The listing builds one solid part. Answer for the finished solid, in the listing's coordinates (mm). A direction names the side the tool comes from. Round coordinates to 2 decimals unless told otherwise and drop trailing zeros. Loops run counter-clockwise (first coordinate to the right, second up) from the corner with the lowest first, then second, coordinate; pieces in that order, holes last. Notation, with made-up numbers: (70.25, -14.75) -> (89.25, -14.75) arc R30 ccw to (89.25, 24.25) -> close; hole circle Ø11 at (80.5, -34). An arc over 180 degrees is marked (long way). Write each question's results on one line, items separated by ' | '. Start each with the question number.
from build123d import *

# Parameters (mm, degrees)
F0_R     = 1
F0_R_2   = 2
F1_DEPTH = 1
F2_R     = 1
F3_DEPTH = 1
F4_SIZE  = 4
F5_SIZE  = 5
F6_R     = 1.5


with BuildPart() as f1:
    # F0 (on Top) → F1 (new body)
    with BuildSketch(Plane.XY):
        with BuildLine():
            Line((-6.25, 2.5), (-6.25, 0))
            ThreePointArc((-6.25, 0), (0, -6.25), (6.25, 0))
            Line((6.25, 0), (6.25, 2.5))
            Line((6.25, 2.5), (-6.25, 2.5))
        make_face()
        with BuildLine():
            ThreePointArc((6.25, 0), (0, -6.25), (-6.25, 0))
            Line((-6.25, 0), (-6.25, 2.5))
            Line((-6.25, 2.5), (-13, 2.5))
            Line((-13, 2.5), (-13, -4.25))
            Line((-13, -4.25), (-10.5, -4.25))
            ThreePointArc((-10.5, -4.25), (-4.25, -10.5), (-10.5, -16.75))
            Line((-10.5, -16.75), (-13, -16.75))
            Line((-13, -16.75), (-13, -32.9777747887))
            Line((-13, -32.9777747887), (13.7, -32.9777747887))
            Line((13.7, -32.9777747887), (13.7, 2.5))
            Line((13.7, 2.5), (6.25, 2.5))
            Line((6.25, 2.5), (6.25, 0))
        make_face()
        with Locations((-10.5, -21)):
            Circle(F0_R, mode=Mode.SUBTRACT)
        with Locations((7.7645713531, -28.9777747887)):
            Circle(F0_R_2, mode=Mode.SUBTRACT)
        with Locations((10.5, -21)):
            Circle(F0_R, mode=Mode.SUBTRACT)
        with Locations((-10.5, 0)):
            Circle(F0_R, mode=Mode.SUBTRACT)
        with Locations((10.5, 0)):
            Circle(F0_R, mode=Mode.SUBTRACT)
    extrude(amount=F1_DEPTH)

    # F2 (on face) → F3 (cut, through all)
    with BuildSketch(Plane.XY.offset(1)):
        Polygon((5.2645713531, -32.9777747887), (-13, -23.5), (-13, -32.9777747887), align=None)
        with BuildLine():
            Line((-13, -16.75), (-13, -18.5))
            Line((-13, -18.5), (8.2, -18.5))
            Line((8.2, -18.5), (8.2, 2.5))
            Line((8.2, 2.5), (-13, 2.5))
            Line((-13, 2.5), (-13, -4.25))
            Line((-13, -4.25), (-10.5, -4.25))
            ThreePointArc((-10.5, -4.25), (-4.25, -10.5), (-10.5, -16.75))
            Line((-10.5, -16.75), (-13, -16.75))
        make_face()
        with Locations((-10.5, 0)):
            Circle(F2_R, mode=Mode.SUBTRACT)
    extrude(amount=-F3_DEPTH, mode=Mode.SUBTRACT)

    # F4
    f4_edges = [f1.edges().sort_by_distance(p)[0] for p in [
        (13.7, -32.977775, 0.5),
    ]]
    chamfer(f4_edges, length=F4_SIZE)

    # F5
    f5_edges = [f1.edges().sort_by_distance(p)[0] for p in [
        (8.2, -18.5, 0.5),
    ]]
    chamfer(f5_edges, length=F5_SIZE)

    # F6
    f6_edges = [f1.edges().sort_by_distance(p)[0] for p in [
        (-13, -23.5, 0.5),
        (5.264571, -32.977775, 0.5),
        (9.7, -32.977775, 0.5),
        (13.7, -28.977775, 0.5),
        (8.2, -13.5, 0.5),
        (3.2, -18.5, 0.5),
        (-13, -18.5, 0.5),
        (13.7, 2.5, 0.5),
        (8.2, 2.5, 0.5),
    ]]
    fillet(f6_edges, radius=F6_R)


solid = f1.part
Item 1: The part is cut by section B-B, the plane x = 10.5. Give the vertices of the cut face in (y, z).
Item 2: The part is cut by section C-C, the plane x = -10.5. Give the vertices of the cut face in (y, z).
Item 3: The part is cut by section A-A, the plane y = 0. Give the vertices of the cut face in (x, z), plus the area to 3 significant figures.
Item 4: For faces 1 (the flat face through (11, 2.5, 0.5)), 2 (the flat face through (8.2, -6, 0.5)), determine the directions among +Z, -Z, +X, -X, +Y, -Y from which every point of the face is accessible in a straight line to the end or side of a thin tool.
Item 5: The part is cut by section D-D, the plane z = 0.55. Give the vertices of the cut face in (x, y), plus the area to 3 significant figures.
Item 6: Determine the mould class of faces 3 (the cylindrical face through (13.6, -28.9, 0.5)), 4 (the flat face through (-3.506, -28.427, 0.507)), 5 (the cylindrical face through (-10.717, -21.976, 0.493)), 6 (the flat face through (7.3, -32.978, 0.5)) for opening direction X: +X half, -X half, draft (parallel to the pull), parting line (faces both ways), or undercut.
Item 7: Each of these flat-tipped pins is pushed along its axis until it touches: pin 1 Ø6.5 at (x, y) = (7.76, -28.98) entering from +Z; pin 2 Ø0.5 at (x, z) = (-6.5, 0.5) entering from +Y; pin 3 Ø0.5 at (y, z) = (-8.5, 0.5) entering from -X. Where does it stop, or does it pass through?
Item 8: Straight lines are drawn through the part: L1, parallel to Y at x = 10.5, z = 0.5; L2, parallel to X at y = -20.5, z = 0.55; L3, parallel to Y at x = 10.75, z = 0.8. For each, find the intervals that lie inside material, in ascending order. Write a range as [from, to].
Report:
1) outline: (-32.18, 0) -> (-22, 0) -> (-22, 1) -> (-32.18, 1) -> close; (-20, 0) -> (-1, 0) -> (-1, 1) -> (-20, 1) -> close; (1, 0) -> (2.5, 0) -> (2.5, 1) -> (1, 1) -> close
2) outline: (-24.8, 0) -> (-22, 0) -> (-22, 1) -> (-24.8, 1) -> close; (-20, 0) -> (-18.5, 0) -> (-18.5, 1) -> (-20, 1) -> close
3) outline: (8.2, 0) -> (9.5, 0) -> (9.5, 1) -> (8.2, 1) -> close; (11.5, 0) -> (13.7, 0) -> (13.7, 1) -> (11.5, 1) -> close | area: 3.50 mm2
4) face 1: +Z, -Z, +X, -X, +Y | face 2: +Z, -Z, -X, +Y
5) outline: (-13, -22.59) arc R1.5 ccw to (-12.19, -23.92) -> (4.94, -32.81) arc R1.5 ccw to (5.63, -32.98) -> (9.08, -32.98) arc R1.5 ccw to (10.14, -32.54) -> (13.26, -29.42) arc R1.5 ccw to (13.7, -28.36) -> (13.7, 1) arc R1.5 ccw to (12.2, 2.5) -> (9.7, 2.5) arc R1.5 ccw to (8.2, 1) -> (8.2, -12.88) arc R1.5 cw to (7.76, -13.94) -> (3.64, -18.06) arc R1.5 cw to (2.58, -18.5) -> (-11.5, -18.5) arc R1.5 ccw to (-13, -20) -> close; hole circle Ø2 at (-10.5, -21); hole circle Ø4 at (7.76, -28.98); hole circle Ø2 at (10.5, -21); hole circle Ø2 at (10.5, 0) | area: 396 mm2
6) face 3: +X half | face 4: -X half | face 5: undercut | face 6: draft
7) pin 1: stops at z = 1 | pin 2: stops at y = -18.5 | pin 3: stops at x = 8.2
8) L1: y = [-32.18, -22], [-20, -1], [1, 2.5] | L2: x = [-13, -11.37], [-9.63, 9.63], [11.37, 13.7] | L3: y = [-31.93, -21.97], [-20.03, -0.97], [0.97, 2.5]
